```python
from build123d import *

# Parameters (mm, degrees)
SKETCH1_R           = 45
SKETCH1_R_2         = 37.5
BOSS_EXTRUDE1_DEPTH = 35
SKETCH2_R           = 42.5
SKETCH2_R_2         = 32.5
EXTRUDE_THIN1_DEPTH = 15
SKETCH3_R           = 1.5
CUT_EXTRUDE1_DEPTH  = 95.604439642
CIRPATTERN1_COUNT   = 8


with BuildPart() as part:
    # Sketch1 → Boss-Extrude1 (new, symmetric)
    with BuildSketch(Plane(origin=(0, 0, 0), x_dir=(1, 0, 0), z_dir=(0, 1, 0))):
        with Locations(Location((0, 0, 0), (0, 0, 270))):
            Circle(SKETCH1_R)
        with Locations(Location((0, 0, 0), (0, 0, 270))):
            Circle(SKETCH1_R_2, mode=Mode.SUBTRACT)
    extrude(amount=BOSS_EXTRUDE1_DEPTH, both=True)

    # Sketch2 → Extrude-Thin1 (add, symmetric)
    with BuildSketch(Plane(origin=(0, 0, 0), x_dir=(1, 0, 0), z_dir=(0, 1, 0))):
        Circle(SKETCH2_R)
        Circle(SKETCH2_R_2, mode=Mode.SUBTRACT)
    extrude(amount=EXTRUDE_THIN1_DEPTH, both=True)

    # Sketch3 → Cut-Extrude1 (cut, through all)
    with BuildSketch(Plane(origin=(0, 35, 0), x_dir=(1, 0, 0), z_dir=(0, 1, 0))):
        with Locations(Location((0, 42, 0), (0, 0, 270))):
            Circle(SKETCH3_R)
    cut_extrude1 = extrude(amount=-CUT_EXTRUDE1_DEPTH, mode=Mode.SUBTRACT)

    # CirPattern1: Cut-Extrude1 ×8 about axis
    cirpattern1_axis = Axis((0, 0, 0), (0, 1, 0))
    for i in range(1, CIRPATTERN1_COUNT):
        add(cut_extrude1.rotate(cirpattern1_axis, i * 360 / CIRPATTERN1_COUNT), mode=Mode.SUBTRACT)


solid = part.part
```
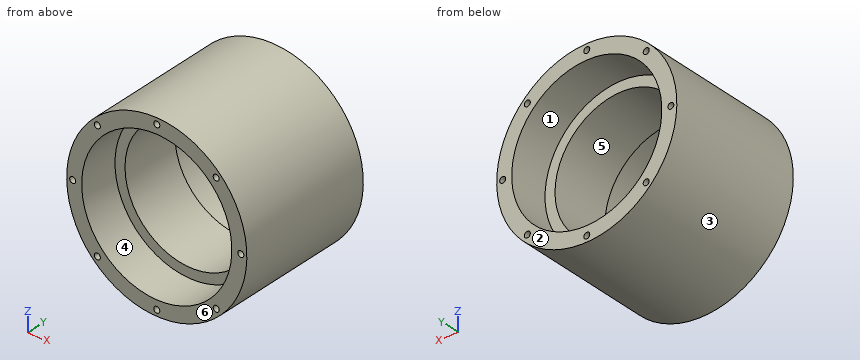
The model under review builds one solid part; all positions refer to its coordinate system, in mm. Face numbers are marked on the shaded views. A direction names the side the tool comes from. Coordinates: 2 decimals unless noted, no trailing zeros. Write each loop counter-clockwise with the first axis right and the second up, starting at its lowest first coordinate (ties: lowest second). Pieces come first, ordered by that corner, then holes.
1) We need section A-A on z = 0. State the section outline as (x, y) points, then the cut area to 3 significant figures.
2) We need section C-C on x = 0. State the section outline as (y, z) points, then the cut area to 3 significant figures.
3) To check wall thickness, follow probe 1 along Y at (x, z) = (-22, 26.5); probe 2 along Z at (x, y) = (-7, -18); probe 3 along Z at (x, y) = (-13, 3.5). State the ranges of each line that lie inside material, in increasing order.
4) Clearance check with flat-ended pins moving along their axes: pin 1 Ø3 at (x, z) = (-32, -2.5) entering from +Y; pin 2 Ø6 at (x, z) = (-28.5, -35.5) entering from +Y; pin 3 Ø2 at (y, z) = (15, -17.5) entering from -X; pin 4 Ø1.5 at (y, z) = (13.5, -30.5) entering from -X. State where each tip first meets the part, or that it passes through.
5) Machinability: for the marked faces 1 and 2, which of the approach directions +Z, -Z, +X, -X, +Y, -Y give a long, thin tool a straight path to every point of the face, cutting with its end or side? Answer none if there is none.
6) We need section D-D on y = 19. Count the separate pieces of the cut face and the enclosed holes in it, then the cut area to 3 significant figures.
7) We need section B-B on x = -13. State the section outline as (y, z) points.
8) The part is to be moulded in two halves that separate along X. For the marked faces 3, 4, 5 and 6, say which applies: pulls with the +X half, pulls with the -X half, needs draft (parallel to the pull), parting line crosses it, or undercut.
Answer list:
1. outline: (-45, -35) - (-43.5, -35) - (-43.5, 35) - (-45, 35) - close; (-40.5, -35) - (-37.5, -35) - (-37.5, -15) - (-32.5, -15) - (-32.5, 15) - (-37.5, 15) - (-37.5, 35) - (-40.5, 35) - close; (32.5, -15) - (37.5, -15) - (37.5, -35) - (40.5, -35) - (40.5, 35) - (37.5, 35) - (37.5, 15) - (32.5, 15) - close; (43.5, -35) - (45, -35) - (45, 35) - (43.5, 35) - close
1. area: 930 mm2
2. outline: (-35, -45) - (35, -45) - (35, -43.5) - (-35, -43.5) - close; (-35, -40.5) - (35, -40.5) - (35, -37.5) - (15, -37.5) - (15, -32.5) - (-15, -32.5) - (-15, -37.5) - (-35, -37.5) - close; (-35, 37.5) - (-15, 37.5) - (-15, 32.5) - (15, 32.5) - (15, 37.5) - (35, 37.5) - (35, 40.5) - (-35, 40.5) - close; (-35, 43.5) - (35, 43.5) - (35, 45) - (-35, 45) - close
2. area: 930 mm2
3. probe 1: y = -15 to 15
3. probe 2: z = -44.45 to -36.84, 36.84 to 44.45
3. probe 3: z = -43.08 to -29.79, 29.79 to 43.08
4. pin 1: stops at y = 15
4. pin 2: stops at y = 35
4. pin 3: stops at x = -41.87
4. pin 4: stops at x = -33.76
5. face 1: +Y
5. face 2: +Z, -Z, +X, -X, +Y
6. separate pieces: 1
6. enclosed holes: 9
6. area: 1,890 mm2
7. outline: (-35, -43.08) - (35, -43.08) - (35, -35.17) - (15, -35.17) - (15, -29.79) - (-15, -29.79) - (-15, -35.17) - (-35, -35.17) - close; (-35, 35.17) - (-15, 35.17) - (-15, 29.79) - (15, 29.79) - (15, 35.17) - (35, 35.17) - (35, 43.08) - (-35, 43.08) - close
8. face 3: parting line crosses it
8. face 4: undercut
8. face 5: undercut
8. face 6: needs draft
